```python
from build123d import *

# Parameters (mm, degrees)
F1_DEPTH = 24
F3_DEPTH = 23
F4_R     = 1.7859375
F5_DEPTH = 25
F7_DEPTH = 3
F8_R     = 1.25
F9_DEPTH = 5
F10_R    = 7


with BuildPart() as f1:
    # F0 (on Top) → F1 (new body)
    with BuildSketch(Plane.XY):
        Polygon((-15, -10), (15, -10), (15, 0), (15, 10), (15, 14), (-15, 14), (-15, 10), (-15, 0), align=None)
    extrude(amount=F1_DEPTH)

    # F2 (on Top) → F3 (cut)
    with BuildSketch(Plane.XY):
        with BuildLine():
            ThreePointArc((-8.2138157895, 0.7718355891), (-8.0544419216, 0.4004520472), (-8, 0))
            ThreePointArc((-8, 0), (-8.0544419216, -0.4004520472), (-8.2138157895, -0.7718355891))
            ThreePointArc((-8.2138157895, -0.7718355891), (0, -8.25), (8.2138157895, -0.7718355891))
            ThreePointArc((8.2138157895, -0.7718355891), (8, 0), (8.2138157895, 0.7718355891))
            ThreePointArc((8.2138157895, 0.7718355891), (0, 8.25), (-8.2138157895, 0.7718355891))
        make_face()
        with BuildLine():
            ThreePointArc((-8.2138157895, -0.7718355891), (-8.25, 0), (-8.2138157895, 0.7718355891))
            ThreePointArc((-8.2138157895, 0.7718355891), (-11, 0), (-8.2138157895, -0.7718355891))
        make_face()
        with BuildLine():
            ThreePointArc((-8.2138157895, -0.7718355891), (-8.0544419216, -0.4004520472), (-8, 0))
            ThreePointArc((-8, 0), (-8.0544419216, 0.4004520472), (-8.2138157895, 0.7718355891))
            ThreePointArc((-8.2138157895, 0.7718355891), (-8.25, 0), (-8.2138157895, -0.7718355891))
        make_face()
        with BuildLine():
            ThreePointArc((8.25, 0), (8.2409489825, 0.3863416473), (8.2138157895, 0.7718355891))
            ThreePointArc((8.2138157895, 0.7718355891), (8, 0), (8.2138157895, -0.7718355891))
            ThreePointArc((8.2138157895, -0.7718355891), (8.2409489825, -0.3863416473), (8.25, 0))
        make_face()
        with BuildLine():
            ThreePointArc((11, 0), (9.9004520472, 1.4455580784), (8.2138157895, 0.7718355891))
            ThreePointArc((8.2138157895, 0.7718355891), (8.2409489825, 0.3863416473), (8.25, 0))
            ThreePointArc((8.25, 0), (8.2409489825, -0.3863416473), (8.2138157895, -0.7718355891))
            ThreePointArc((8.2138157895, -0.7718355891), (9.9004520472, -1.4455580784), (11, 0))
        make_face()
    extrude(amount=F3_DEPTH, mode=Mode.SUBTRACT)

    # F4 (on face) → F5 (cut)
    with BuildSketch(Plane(origin=(0, 0, 23), x_dir=(1, 0, 0), z_dir=(0, 0, -1))):
        Circle(F4_R)
    extrude(amount=-F5_DEPTH, mode=Mode.SUBTRACT)

    # F6 (on face) → F7 (cut)
    with BuildSketch(Plane(origin=(0, 0, 0), x_dir=(1, 0, 0), z_dir=(0, 0, -1))):
        with BuildLine():
            ThreePointArc((8.8741196746, -9.5), (11.9240000791, -5.1786312974), (13, 0))
            ThreePointArc((13, 0), (11.9240000791, 5.1786312974), (8.8741196746, 9.5))
            Line((8.8741196746, 9.5), (8.8741196746, 1.3631851739))
            ThreePointArc((8.8741196746, 1.3631851739), (11, 0), (8.8741196746, -1.3631851739))
            Line((8.8741196746, -1.3631851739), (8.8741196746, -9.5))
        make_face()
        with BuildLine():
            Line((8.8741196746, 1.3631851739), (8.8741196746, 9.5))
            Line((8.8741196746, 9.5), (-8.8741196746, 9.5))
            Line((-8.8741196746, 9.5), (-8.8741196746, 1.3631851739))
            ThreePointArc((-8.8741196746, 1.3631851739), (-8.4992896122, 1.1173981921), (-8.2138157895, 0.7718355891))
            ThreePointArc((-8.2138157895, 0.7718355891), (0, 8.25), (8.2138157895, 0.7718355891))
            ThreePointArc((8.2138157895, 0.7718355891), (8.4992896122, 1.1173981921), (8.8741196746, 1.3631851739))
        make_face()
        with BuildLine():
            Line((-8.8741196746, -9.5), (8.8741196746, -9.5))
            Line((8.8741196746, -9.5), (8.8741196746, -1.3631851739))
            ThreePointArc((8.8741196746, -1.3631851739), (8.4992896122, -1.1173981921), (8.2138157895, -0.7718355891))
            ThreePointArc((8.2138157895, -0.7718355891), (0, -8.25), (-8.2138157895, -0.7718355891))
            ThreePointArc((-8.2138157895, -0.7718355891), (-8.4992896122, -1.1173981921), (-8.8741196746, -1.3631851739))
            Line((-8.8741196746, -1.3631851739), (-8.8741196746, -9.5))
        make_face()
        with BuildLine():
            Line((-8.8741196746, 1.3631851739), (-8.8741196746, 9.5))
            ThreePointArc((-8.8741196746, 9.5), (-13, 0), (-8.8741196746, -9.5))
            Line((-8.8741196746, -9.5), (-8.8741196746, -1.3631851739))
            ThreePointArc((-8.8741196746, -1.3631851739), (-11, 0), (-8.8741196746, 1.3631851739))
        make_face()
        with BuildLine():
            ThreePointArc((8.8741196746, -1.3631851739), (11, 0), (8.8741196746, 1.3631851739))
            Line((8.8741196746, 1.3631851739), (8.8741196746, -1.3631851739))
        make_face()
        with BuildLine():
            Line((8.8741196746, -1.3631851739), (8.8741196746, 1.3631851739))
            ThreePointArc((8.8741196746, 1.3631851739), (8.4992896122, 1.1173981921), (8.2138157895, 0.7718355891))
            ThreePointArc((8.2138157895, 0.7718355891), (0, 8.25), (-8.2138157895, 0.7718355891))
            ThreePointArc((-8.2138157895, 0.7718355891), (-8.4992896122, 1.1173981921), (-8.8741196746, 1.3631851739))
            Line((-8.8741196746, 1.3631851739), (-8.8741196746, -1.3631851739))
            ThreePointArc((-8.8741196746, -1.3631851739), (-8.4992896122, -1.1173981921), (-8.2138157895, -0.7718355891))
            ThreePointArc((-8.2138157895, -0.7718355891), (0, -8.25), (8.2138157895, -0.7718355891))
            ThreePointArc((8.2138157895, -0.7718355891), (8.4992896122, -1.1173981921), (8.8741196746, -1.3631851739))
        make_face()
        with BuildLine():
            Line((-8.8741196746, -1.3631851739), (-8.8741196746, 1.3631851739))
            ThreePointArc((-8.8741196746, 1.3631851739), (-11, 0), (-8.8741196746, -1.3631851739))
        make_face()
    extrude(amount=-F7_DEPTH, mode=Mode.SUBTRACT)

    # F8 (on face) → F9 (cut)
    with BuildSketch(Plane(origin=(0, 14, 0), x_dir=(-1, 0, 0), z_dir=(0, 1, 0))):
        with Locations((-10, 7)):
            Circle(F8_R)
        with Locations((10, 7)):
            Circle(F8_R)
    extrude(amount=-F9_DEPTH, mode=Mode.SUBTRACT)

    # F10
    f10_edges = [f1.edges().sort_by_distance(p)[0] for p in [
        (-15, -10, 12),
        (15, -10, 12),
    ]]
    fillet(f10_edges, radius=F10_R)


solid = f1.part
```
Design review of the part built by this model. Coordinates are the model's own, in mm. A direction names the side the tool comes from. Round coordinates to 2 decimals unless told otherwise and drop trailing zeros. Write each loop counter-clockwise with the first axis right and the second up, starting at its lowest first coordinate (ties: lowest second). Pieces come first, ordered by that corner, then holes. Notation, with made-up numbers: (-31, 10) -> (-3, 10) arc R22 ccw to (-3, 31) -> close; hole circle Ø9 at (28.25, -22.5). An arc over 180 degrees is marked (long way). Answer in a Markdown table with one row per item.
Q1. Take a section at B-B, the plane z = 7. State the section outline as (x, y) points, then the cut area to 3 significant figures.
The answers:
| item | result |
|---|---|
| outline | (-15, -3) arc R7 ccw to (-8, -10) -> (8, -10) arc R7 ccw to (15, -3) -> (15, 14) -> (11.25, 14) -> (11.25, 9) -> (8.75, 9) -> (8.75, 14) -> (-8.75, 14) -> (-8.75, 9) -> (-11.25, 9) -> (-11.25, 14) -> (-15, 14) -> close; hole (-8.21, -0.77) arc R8.25 ccw to (8.21, -0.77) arc R1.5 ccw (long way) to (8.21, 0.77) arc R8.25 ccw to (-8.21, 0.77) arc R1.5 ccw (long way) to start |
| area | 447 mm² |
Q2. Draft analysis for pull direction X (two halves, no side actions). For faces 4 (the face through (-8.75, 11.54, 7.05)), 5 (the face through (-12.9, -8, 12.2)), 6 (the face through (0, -10, 12)), 7 (the face through (15, 5, 12)), state which applies: +X half, -X half, draft (parallel to the pull), parting line (faces both ways), or undercut.
The answers:
| item | result |
|---|---|
| face 4 | undercut |
| face 5 | -X half |
| face 6 | draft |
| face 7 | +X half |
Q3. For faces 1 (the face through (-0.17, -8.25, 12.86)), 2 (the face through (0, 10, 0)), 3 (the face through (-10, 9, 7)), list the 3-axis set-ups (+Z, -Z, +X, -X, +Y, -Y) from which the entire face can be reached by the end or side of a thin tool; tool diameter is ignored.
The answers:
| item | result |
|---|---|
| face 1 | -Z |
| face 2 | -Z, +X, -X, +Y, -Y |
| face 3 | +Y |
Q4. Take a section at D-D, the plane z = 13.5. State the section outline as (x, y) points.
The answers:
| item | result |
|---|---|
| outline | (-15, -3) arc R7 ccw to (-8, -10) -> (8, -10) arc R7 ccw to (15, -3) -> (15, 14) -> (-15, 14) -> close; hole (-8.21, -0.77) arc R8.25 ccw to (8.21, -0.77) arc R1.5 ccw (long way) to (8.21, 0.77) arc R8.25 ccw to (-8.21, 0.77) arc R1.5 ccw (long way) to start |
Q5. Clearance check with flat-ended pins moving along their axes: pin 1 Ø0.8 at (x, z) = (10, 7.5) entering from +Y; pin 2 Ø13 at (x, y) = (-4, 0.5) entering from -Z; pin 3 Ø1 at (x, y) = (-3, -1) entering from -Z. State where each tip first meets the part, or that it passes through.
The answers:
| item | result |
|---|---|
| pin 1 | y = 9 |
| pin 2 | z = 3 |
| pin 3 | z = 23 |
Q6. To check wall thickness, follow L1, parallel to X at y = 0, z = 13.5; L2, parallel to Y at x = -3.5, z = 2.5; L3, parallel to Y at x = 2, z = 4.25. State the ranges of each line that lie inside material, in increasing order. Write a range as [from, to].
The answers:
| item | result |
|---|---|
| L1 | [-15, -11], [11, 15] |
| L2 | [-10, -9.5], [9.5, 14] |
| L3 | [-10, -8], [8, 14] |
Q7. Take a section at C-C, the plane x = 9.75. State the section outline as (y, z) points, then the cut area to 3 significant figures.
The answers:
| item | result |
|---|---|
| outline | (-9.78, 0) -> (-8.6, 0) -> (-8.6, 3) -> (-1.48, 3) -> (-1.48, 23) -> (1.48, 23) -> (1.48, 3) -> (8.6, 3) -> (8.6, 0) -> (14, 0) -> (14, 5.78) -> (9, 5.78) -> (9, 8.22) -> (14, 8.22) -> (14, 24) -> (-9.78, 24) -> close |
| area | 448 mm² |
Q8. Take a section at A-A, the plane x = 0. State the section outline as (y, z) points, then the cut area to 3 significant figures.
The answers:
| item | result |
|---|---|
| outline | (-10, 0) -> (-9.5, 0) -> (-9.5, 3) -> (-8.25, 3) -> (-8.25, 23) -> (-1.79, 23) -> (-1.79, 24) -> (-10, 24) -> close; (1.79, 23) -> (8.25, 23) -> (8.25, 3) -> (9.5, 3) -> (9.5, 0) -> (14, 0) -> (14, 24) -> (1.79, 24) -> close |
| area | 185 mm² |
